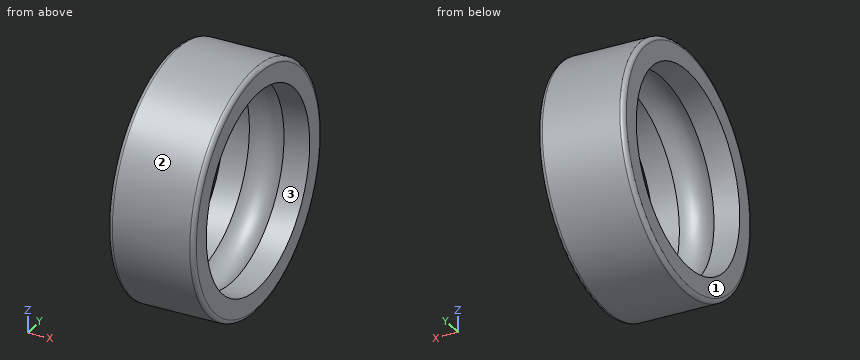
Autodesk Inventor part; units mm, degrees
ref_plane "ip_ot_or_XY" through (0, 0, 0) normal (1, 0, 0) x (0, 0, -1)
ref_plane "ip_ot_or_YZ" through (0, 0, 0) normal (0, 0, -1) x (0, 1, 0)
ref_plane "ip_ot_or_ZX" through (0, 0, 0) normal (0, 1, 0) x (1, 0, 0)
sketch "Sketch_1" plane through (0, 0, 0) normal (0, 0, 1) x (1, 0, 0)
  line L0 (6, 0) -> (0, 0)
  line L1 (0, 6.875) -> (1.793, 6.875)
  arc A0 (4.207, 6.875) -> (1.793, 6.875) centre (3, 5.75) ccw
  line L2 (4.207, 6.875) -> (6, 6.875)
  line L3 (6, 6.875) -> (6, 8.2)
  arc A1 (6, 8.2) -> (5.7, 8.5) centre (5.7, 8.2) ccw
  line L4 (5.7, 8.5) -> (0.3, 8.5)
  arc A2 (0.3, 8.5) -> (0, 8.2) centre (0.3, 8.2) ccw
  line L5 (0, 8.2) -> (0, 6.875)
revolve "Revolution1" add sketch "Sketch_1" angle 360 about axis through (6, 0, 0) along (1, 0, 0)
ref_plane "ip_ot_or_XY" through (0, 0, 0) normal (1, 0, 0) x (0, 0, -1)
ref_plane "ip_ot_or_YZ" through (0, 0, 0) normal (0, 0, -1) x (0, 1, 0)
ref_plane "ip_ot_or_ZX" through (0, 0, 0) normal (0, 1, 0) x (1, 0, 0)
properties part number "606 Outer Ring" material "Steel"
Geometry: final body of the model. Coordinates: model frame, mm. Face numbers are marked on the shaded views. Coordinates: 2 decimals unless noted, no trailing zeros. Write each loop counter-clockwise with the first axis right and the second up, starting at its lowest first coordinate (ties: lowest second). Pieces come first, ordered by that corner, then holes. Notation, with made-up numbers: (-39.5, -22) - (6.5, -22) arc R15 cw to (6.5, -8) - close; hole circle Ø11 at (15, -3). An arc over 180 degrees is marked (long way). Return JSON: item names as keys, results as strings.
Item 1: Line query: L1, parallel to Z at x = 4.85, y = 0 (3 decimals); L2, parallel to Z at x = 2.25, y = -6.5; L3, parallel to X at y = -4.5, z = 5.5. Output: solid intervals per line, ascending.
Completed:
{"L1": "z = -8.5 to -6.875, 6.875 to 8.5", "L2": "z = -5.48 to -3.14, 3.14 to 5.48", "L3": "x = 0 to 2.06, 3.94 to 6"}
Item 2: Pin query (flat end, axial travel): pin 1 Ø8 at (y, z) = (0, 0) entering from -X; pin 2 Ø1.5 at (x, y) = (0.5, -6) entering from -Z. Return the tip coordinate at first contact, or that it passes through.
Completed:
{"pin 1": "passes through", "pin 2": "stops at z = -6.68"}
Item 3: Pull-direction query (Y, two-part tool) for the marked faces 1, 2 and 3; classes: +Y half, -Y half, draft (parallel to the pull), parting line (faces both ways), or undercut.
Completed:
{"face 1": "draft", "face 2": "parting line", "face 3": "undercut"}
Item 4: Section query A-A (y = 0). Output: boundary loops of the cut face in (x, z) (3 decimals), and give its area (3 significant figures).
Completed:
{"outline": "(0, -8.2) arc R0.3 ccw to (0.3, -8.5) - (5.7, -8.5) arc R0.3 ccw to (6, -8.2) - (6, -6.875) - (4.207, -6.875) arc R1.65 cw to (1.793, -6.875) - (0, -6.875) - close; (0, 6.875) - (1.793, 6.875) arc R1.65 cw to (4.207, 6.875) - (6, 6.875) - (6, 8.2) arc R0.3 ccw to (5.7, 8.5) - (0.3, 8.5) arc R0.3 ccw to (0, 8.2) - close", "area": "17.7 mm2"}
Item 5: Section query C-C (x = 4.75). Output: boundary loops of the cut face in (y, z) (3 decimals), and give its area (3 significant figures).
Completed:
{"outline": "circle Ø17 at (0, 0); hole circle Ø13.75 at (0, 0)", "area": "78.5 mm2"}
